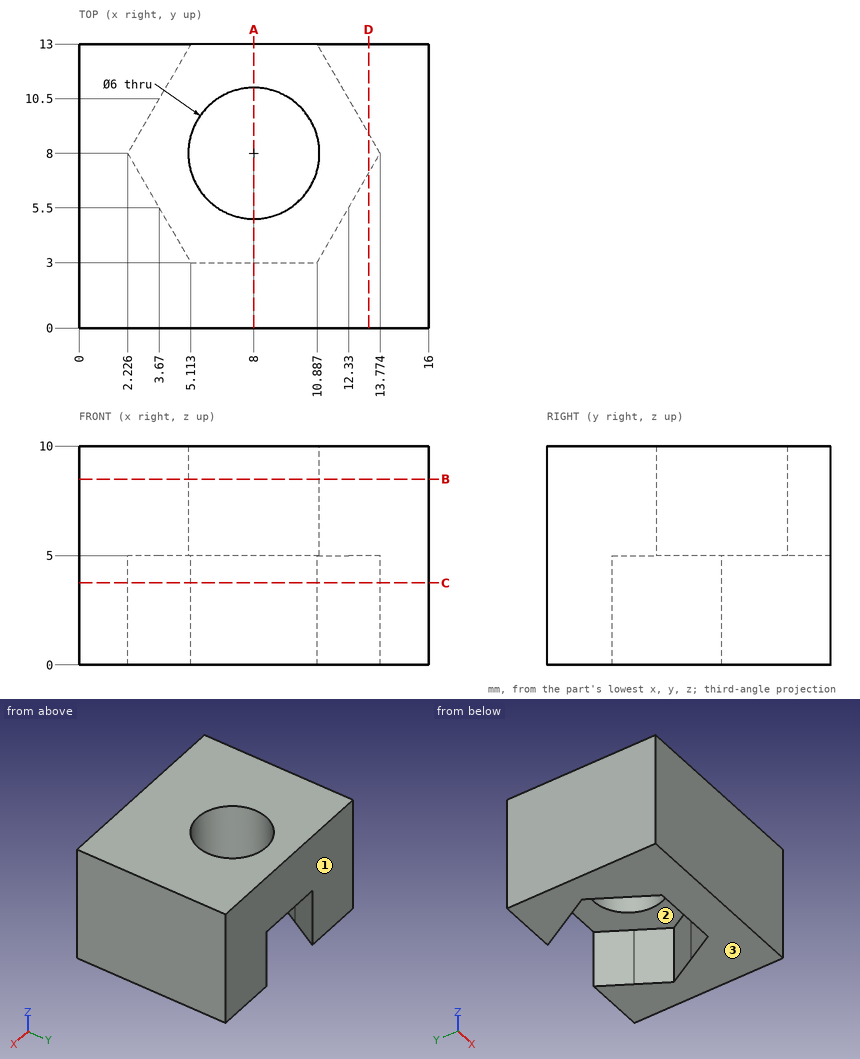
Design review of the part shown in the three views and the two pictorial views. Dimensions are in mm from the part's minimum x, y and z. Round coordinates to 2 decimals unless told otherwise and drop trailing zeros. Write each loop counter-clockwise with the first axis right and the second up, starting at its lowest first coordinate (ties: lowest second). Pieces come first, ordered by that corner, then holes. Notation, with made-up numbers: (10, -34) - (24, -34) arc R24 cw to (24, -15) - close; hole circle Ø1 at (29.5, 0). An arc over 180 degrees is marked (long way). Return JSON: item names as keys, results as strings. Group by question number.
Item 1: The part is to be moulded in two halves that separate along Y. For the marked faces 1, 2 and 3, say which applies: pulls with the +Y half, pulls with the -Y half, needs draft (parallel to the pull), parting line crosses it, or undercut.
Item 2: We need section B-B on z = 8.5. Write out the cut boundary in (x, y), and give its area (3 significant figures).
Item 3: We need section C-C on z = 3.75. Write out the cut boundary in (x, y).
Item 4: For probe 1 along Y at (x, z) = (8, 6.85); probe 2 along Z at (x, y) = (11.75, 9.5); probe 3 along Y at (x, z) = (8.75, 8.5) (1 decimal), list the stretches that pass through material, from the lowest coordinate up. Write a range as [from, to].
Item 5: We need section A-A on x = 8. Write out the cut boundary in (y, z).
Item 6: We need section D-D on x = 13.25. Write out the cut boundary in (y, z), and give its area (3 significant figures).
Item 7: Insertion check: P1, Ø2.5, axis at x = 8.5, z = 3.5, coming from the +Y side. The pin has a flat end and moves straight along its axis. Give the tip position at first contact, or say it passes through.
Model answer:
{
 "1": {"face 1": "pulls with the +Y half", "face 2": "undercut", "face 3": "needs draft"},
 "2": {"outline": "(0, 0) - (16, 0) - (16, 13) - (0, 13) - close; hole circle Ø6 at (8, 8)", "area": "180 mm²"},
 "3": {"outline": "(0, 0) - (16, 0) - (16, 13) - (10.89, 13) - (12.33, 10.5) - (13.77, 8) - (12.33, 5.5) - (10.89, 3) - (5.11, 3) - (3.67, 5.5) - (2.23, 8) - (3.67, 10.5) - (5.11, 13) - (0, 13) - close"},
 "4": {"probe 1": "y = [0, 5], [11, 13]", "probe 2": "z = [5, 10]", "probe 3": "y = [0, 5.1], [10.9, 13]"},
 "5": {"outline": "(0, 0) - (3, 0) - (3, 5) - (5, 5) - (5, 10) - (0, 10) - close; (11, 5) - (13, 5) - (13, 10) - (11, 10) - close"},
 "6": {"outline": "(0, 0) - (7.09, 0) - (7.09, 5) - (8.91, 5) - (8.91, 0) - (13, 0) - (13, 10) - (0, 10) - close", "area": "121 mm²"},
 "7": {"P1": "stops at y = 3"}
}
